Build history of the part. All positions in model axes, mm. Coordinates: 2 decimals unless noted, no trailing zeros. Write each loop counter-clockwise with the first axis right and the second up, starting at its lowest first coordinate (ties: lowest second). Pieces come first, ordered by that corner, then holes.
from build123d import *

# Parameters (mm, degrees)
F1_ANGLE = 30


with BuildPart() as f1:
    # F0 (on Front) → F1 (revolve)
    with BuildSketch(Plane.XZ):
        Polygon((0, -85.375826), (0, 0), (-14.692988, 41.624174), (-32.847719, 41.624174), (-46.950776, 0), (-66.58428, 41.624174), (-76.2, 41.624174), (-76.2, -85.375826), align=None)
    revolve(axis=Axis((0, 0, -21.875826), (0, 0, -1)), revolution_arc=F1_ANGLE)


solid = f1.part
(1) Two-plate mould, pull along X, no slides. Class faces 1 (the conical face through (-38.673, 10.211, 20.521)), 2 (the cylindrical face through (-73.675, 19.452, -22.765)), 3 (the flat face through (-39, 0, -21)), 4 (the conical face through (-55.02, 14.527, 21.103)): pulls with the +X half, pulls with the -X half, needs draft (parallel to the pull), parting line crosses it, or undercut.
(2) Probe L1, parallel to X at y = 10, z = 31.5; L2, parallel to X at y = 12.5, z = -75; L3, parallel to X at y = 6, z = 22.5. List the from-to ranges inside material, lowest first.
(3) Slice it at A-A, the plane z = 8. List the corners of the cut face in (x, y).
(4) Slice it at C-C, the plane x = -16.5. List the corners of the cut face in (y, z).
(5) Slice it at B-B, the plane z = -62.5. List the corners of the cut face in (x, y).
(6) Flat gauge pins, fed straight in: P1, Ø5, axis at x = -66.5, z = -71.5, coming from the -Y side; P2, Ø10, axis at y = 11, z = 15, coming from the +X side; P3, Ø3, axis at y = 28, z = -58.5, coming from the -X side; P4, Ø12, axis at y = 18.5, z = -26.5, coming from the +X side. Where does each tip first touch, or does it go through?
Results:
1. face 1: undercut
1. face 2: pulls with the -X half
1. face 3: needs draft
1. face 4: undercut
2. L1: x = -75.54 to -60.99, -34.87 to -17.32
2. L2: x = -75.17 to -21.65
2. L3: x = -75.96 to -57.25, -38.87 to -10.39
3. outline: (-76.2, 0) - (-50.72, 0) arc R50.72 cw to (-43.93, 25.36) - (-65.99, 38.1) arc R76.2 ccw to start; (-44.24, 0) - (-2.82, 0) arc R2.82 cw to (-2.45, 1.41) - (-38.31, 22.12) arc R44.24 ccw to start
4. outline: (0, -85.38) - (9.53, -85.38) - (9.53, 41.62) - (0, 41.62) - close
5. outline: (-76.2, 0) - (0, 0) - (-65.99, 38.1) arc R76.2 ccw to start
6. P1: stops at y = 0
6. P2: stops at x = -10.39
6. P3: stops at x = -71.44
6. P4: stops at x = -21.65
